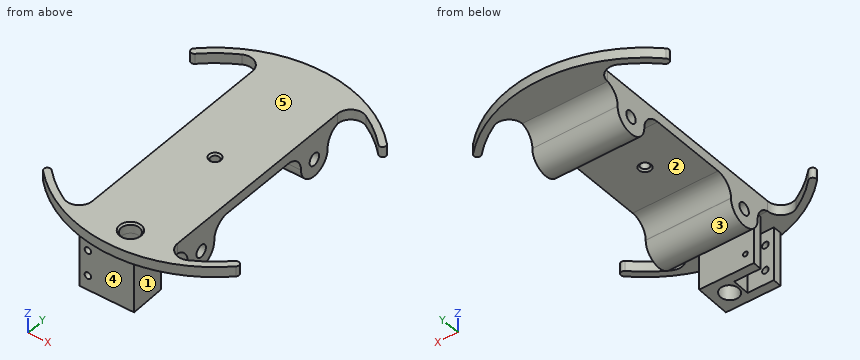
```python
from build123d import *

# Parameters (mm, degrees)
MAIN_BODY_DEPTH                 = 3.81
BOSSES_FOR_SCREWS_DEPTH         = 31.75
F_8_CLEARANCE_HOLE_FOR_SCREWS_D = 4.4958
SWITCH_HOLDER_BODY_REACH        = 65.711
SKETCH19_R                      = 3.3782
F_1_4_QR_PIN_HOLE_D             = 6.7564
F_1_4_QR_PIN_HOLE_CSINK_D       = 8.0264
F_1_4_QR_PIN_HOLE_CSINK_ANGLE   = 90
SKETCH25_R                      = 1.862
PLUNGER_HOLE_DEPTH              = 2.54
SKETCH33_W                      = 6.4
SKETCH33_H                      = 6.4
SWITCH_BODY_CLEARANCE_DEPTH     = 0.65024
F_2_CLEARANCE_HOLE1_D           = 2.4384
F_2_CLEARANCE_HOLE1_DEPTH       = 3.175
TAP_DRILL_FOR_2_56_TAP1_D       = 1.778
TAP_DRILL_FOR_2_56_TAP1_DEPTH   = 12.7


with BuildPart() as part:
    # Sketch3 → Main Body (new body)
    with BuildSketch(Plane.XY):
        with BuildLine():
            Line((-15.875, -38.1), (-15.875, 38.1))
            ThreePointArc((-15.875, 38.1), (-18.260491841, 42.291797068), (-23.082694008, 42.38179842))
            ThreePointArc((-23.082694008, 42.38179842), (-28.900226452, 38.649767283), (-34.12497326, 34.12497326))
            ThreePointArc((-34.12497326, 34.12497326), (-35.921024484, 34.12497326), (-35.921024484, 35.921024484))
            ThreePointArc((-35.921024484, 35.921024484), (0, 50.8), (35.921024484, 35.921024484))
            ThreePointArc((35.921024484, 35.921024484), (35.921024484, 34.12497326), (34.12497326, 34.12497326))
            ThreePointArc((34.12497326, 34.12497326), (28.900226452, 38.649767283), (23.082694008, 42.38179842))
            ThreePointArc((23.082694008, 42.38179842), (18.260491841, 42.291797068), (15.875, 38.1))
            Line((15.875, 38.1), (15.875, -38.1))
            ThreePointArc((15.875, -38.1), (18.260491841, -42.291797068), (23.082694008, -42.38179842))
            ThreePointArc((23.082694008, -42.38179842), (28.900226452, -38.649767283), (34.12497326, -34.12497326))
            ThreePointArc((34.12497326, -34.12497326), (35.921024484, -34.12497326), (35.921024484, -35.921024484))
            ThreePointArc((35.921024484, -35.921024484), (0, -50.8), (-35.921024484, -35.921024484))
            ThreePointArc((-35.921024484, -35.921024484), (-35.921024484, -34.12497326), (-34.12497326, -34.12497326))
            ThreePointArc((-34.12497326, -34.12497326), (-28.900226452, -38.649767283), (-23.082694008, -42.38179842))
            ThreePointArc((-23.082694008, -42.38179842), (-18.260491841, -42.291797068), (-15.875, -38.1))
        make_face()
    extrude(amount=MAIN_BODY_DEPTH)

    # Sketch5 → Bosses for screws (add)
    with BuildSketch(Plane(origin=(15.875, 0, 0), x_dir=(0, 0, -1), z_dir=(1, 0, 0))):
        with BuildLine():
            Line((0, 38.1), (0, 26.99385))
            Line((0, 26.99385), (0, 14.29385))
            ThreePointArc((0, 14.29385), (1.86498297, 18.77886703), (6.35, 20.64385))
            ThreePointArc((6.35, 20.64385), (12.699998494, 26.998224058), (6.341251887, 33.343843974))
            ThreePointArc((6.341251887, 33.343843974), (2.338844583, 34.612930799), (0, 38.1))
        make_face()
        with BuildLine():
            ThreePointArc((6.261703048, -20.644463916), (1.864650947, -18.840779739), (0, -14.469233029))
            Line((0, -14.469233029), (0, -26.99385))
            Line((0, -26.99385), (0, -38.1))
            ThreePointArc((0, -38.1), (2.217611083, -34.670801888), (6.077775616, -33.338012189))
            ThreePointArc((6.077775616, -33.338012189), (6.213919542, -33.33945129), (6.35, -33.34385))
            ThreePointArc((6.35, -33.34385), (12.7, -26.99385), (6.35, -20.64385))
            ThreePointArc((6.35, -20.64385), (6.305852606, -20.644312569), (6.261703048, -20.644463916))
        make_face()
    extrude(amount=-BOSSES_FOR_SCREWS_DEPTH)

    # #8 Clearance Hole for screws (through all)
    with Locations(Plane(origin=(15.875, 0, 0), x_dir=(0, 0, -1), z_dir=(1, 0, 0))):
        with Locations((6.35, 26.99385), (6.35, -26.893399733)):
            Hole(F_8_CLEARANCE_HOLE_FOR_SCREWS_D / 2)

    # Sketch10 → 1/8 (0.125) Diameter let down hole (revolve, cut)
    with BuildSketch(Plane.YZ):
        Polygon((0, 0), (0, 3.81), (2.2225, 3.81), (1.5875, 3.175), (1.5875, 0.635), (2.2225, 0), align=None)
    revolve(axis=Axis((0, 0, -6.35), (0, 0, 1)), mode=Mode.SUBTRACT)

    # Switch holder body: up to this plane
    switch_holder_body_end = Plane(origin=(-3.297630422, -38.686979812, -19.719207275), z_dir=(0.008390733100517729, 0.03489949670250099, -0.9993556027400597))
    # Sketch19 → Switch holder body (add, up to the surface)
    with BuildSketch(Plane(origin=(0, 0, 0), x_dir=(-1, 0, 0), z_dir=(0, 0, -1)), mode=Mode.PRIVATE) as switch_holder_body_sk1:
        Polygon((12.7, -38.735), (2.921, -38.735), (2.921, -45.085), (12.7, -45.085), (12.7, -48.26), (-7.62, -48.26), (-7.62, -35.56), (12.7, -35.56), align=None)
        with Locations(Location((-1.27, -41.91, 0), (0, 0, 103.518789087))):
            Circle(SKETCH19_R, mode=Mode.SUBTRACT)
    switch_holder_body_tool1 = split(extrude(switch_holder_body_sk1.sketch, amount=SWITCH_HOLDER_BODY_REACH, mode=Mode.PRIVATE), bisect_by=switch_holder_body_end, keep=Keep.BOTH, mode=Mode.PRIVATE)
    add(switch_holder_body_tool1.solids().sort_by_distance((-7.8105, -38.495377, 0))[0])

    # 1/4 QR pin hole (through all)
    with Locations(Plane.XY.offset(3.81)):
        with Locations((1.27, -41.91)):
            CounterSinkHole(F_1_4_QR_PIN_HOLE_D / 2, F_1_4_QR_PIN_HOLE_CSINK_D / 2, counter_sink_angle=F_1_4_QR_PIN_HOLE_CSINK_ANGLE)

    # Sketch25 → plunger hole (cut)
    with BuildSketch(Plane.ZY.offset(2.921)):
        with Locations(Location((-7.285, -41.935, 0), (0, 0, 270))):
            Circle(SKETCH25_R)
    extrude(amount=-PLUNGER_HOLE_DEPTH, mode=Mode.SUBTRACT)

    # Sketch33 → switch body clearance (cut)
    with BuildSketch(Plane.ZY.offset(2.921)):
        with Locations((-7.285, -41.935)):
            Rectangle(SKETCH33_W, SKETCH33_H)
    extrude(amount=-SWITCH_BODY_CLEARANCE_DEPTH, mode=Mode.SUBTRACT)

    # #2 Clearance Hole1
    with Locations(Plane(origin=(0, -48.26, 0), x_dir=(-1, 0, 0), z_dir=(0, -1, 0))):
        with Locations((9.571, 14.7), (9.571, 5.2)):
            Hole(F_2_CLEARANCE_HOLE1_D / 2, depth=F_2_CLEARANCE_HOLE1_DEPTH)

    # Tap Drill for #2-56 Tap1
    with Locations(Plane(origin=(0, -48.26, 0), x_dir=(-1, 0, 0), z_dir=(0, -1, 0))):
        with Locations((9.571, 14.7), (9.571, 5.2)):
            Hole(TAP_DRILL_FOR_2_56_TAP1_D / 2, depth=TAP_DRILL_FOR_2_56_TAP1_DEPTH)


solid = part.part
```
CAD build for the part. Positions are in the model's coordinates, mm. Face numbers are marked on the shaded views. A direction names the side the tool comes from. Give positions to 0.01 mm unless a question says otherwise; leave off trailing zeros. Order: outer loops, then holes, each group sorted by start corner. A loop starts at its lowest first (then second) coordinate and runs counter-clockwise, first axis right, second up.
(1) Drill centre lines: L1, parallel to Y at x = -11, z = -17 (3 decimals); L2, parallel to Y at x = -4, z = -3 (3 decimals); L3, parallel to Y at x = 1, z = -17.5. Where is each one in solid material? Low to high.
(2) Mould opens along Y. For the marked faces 3, 4 and 5 say: released by +Y, released by -Y, zero draft, split by the parting line, or undercut.
(3) Tool access for the marked faces 1 and 2: list every direction of +Z, -Z, +X, -X, +Y, -Y with a clear straight run to the whole face (end or side of a thin tool).
(4) Saw through at D-D, the plane x = -18.5. Give the cut face in (y, z).
(5) Flat gauge pins, fed straight in: pin 1 (5 mm diameter, centred on y = -40.5, z = -7.5, fed in from -X); pin 2 (9 mm diameter, centred on x = -6, z = -14, fed in from +Y); pin 3 (12 mm diameter, centred on x = 19, z = 0, fed in from +Y). Where does each tip first touch, or does it go through?
(6) Saw through at A-A, the plane x = -26.5. Give the cut face in (y, z).
(7) Saw through at C-C, the plane y = -10. Give the cut face in (x, z) (3 decimals).
(8) Saw through at B-B, the plane x = 0. State how many separate pieces and enclosed holes the cut face has, then the cut area to 3 significant figures.
Results found:
1. L1: y = -48.26 to -45.085, -38.735 to -35.56
1. L2: y = -48.26 to -45.085, -38.735 to -35.56, -34.148 to -19.728, 19.681 to 34.179
1. L3: y = -48.26 to -45.28, -38.54 to -35.56
2. face 3: undercut
2. face 4: released by -Y
2. face 5: zero draft
3. face 1: -Z, +X, -Y
3. face 2: -Z, +X, -X
4. outline: (-47.31, 0) - (-42.43, 0) - (-42.43, 3.81) - (-47.31, 3.81) - close; (42.43, 0) - (47.31, 0) - (47.31, 3.81) - (42.43, 3.81) - close
5. pin 1: stops at x = -12.7
5. pin 2: stops at y = 32.51
5. pin 3: stops at y = 49.11
6. outline: (-43.34, 0) - (-40.33, 0) - (-40.33, 3.81) - (-43.34, 3.81) - close; (40.33, 0) - (43.34, 0) - (43.34, 3.81) - (40.33, 3.81) - close
7. outline: (-15.875, 0) - (15.875, 0) - (15.875, 3.81) - (-15.875, 3.81) - close
8. separate pieces: 3
8. enclosed holes: 2
8. area: 764 mm2
